For this review, take the finished solid that the model builds, in its own axes (mm). Face numbers are marked on the shaded views. A direction names the side the tool comes from. Coordinates: 2 decimals unless noted, no trailing zeros. Loops run counter-clockwise (first coordinate to the right, second up) from the corner with the lowest first, then second, coordinate; pieces in that order, holes last. Notation, with made-up numbers: (3.25, -38.75) - (42.25, -38.75) arc R20 ccw to (42.25, -6.75) - close; hole circle Ø11 at (86, -16). An arc over 180 degrees is marked (long way). Use one line per item in the form item = value. Start each with the question number.
1. Draft analysis for pull direction X (two halves, no side actions). For the marked faces 1, 2 and 3, state which applies: +X half, -X half, draft (parallel to the pull), parting line (faces both ways), or undercut.
2. For pin 1 Ø4.5 at (x, y) = (63, 0) entering from +Z; pin 2 Ø4 at (x, z) = (55.5, -1) entering from -Y; pin 3 Ø4 at (x, y) = (56.5, 2.5) entering from -Z, all flat-tipped, find the tip position at first contact; note any pin that passes through.
3. Add section B-B on x = 18. Give the boundary of the cut face in (y, z), and give its area (3 significant figures).
4. To check wall thickness, follow probe 1 along X at (y, z) = (0, 3.2); probe 2 along Z at (x, y) = (22.5, -5); probe 3 along X at (y, z) = (0, -1.25). State the ranges of each line that lie inside material, in increasing order.
5. Machinability: for the marked faces 4 and 5, which of the approach directions +Z, -Z, +X, -X, +Y, -Y give a long, thin tool a straight path to every point of the face, cutting with its end or side? Answer none if there is none.
6. Add section A-A on y = 0. Count the separate pieces of the cut face and the enclosed holes in it, and give its area (3 significant figures).
```python
from build123d import *

# Parameters (mm, degrees)
SKIZZE1_W                            = 63
SKIZZE1_H                            = 6
SKIZZE2_W                            = 18
SKIZZE2_H                            = 14
AUFSATZ_LINEAR_AUSTRAGEN1_DEPTH      = 9
SCHNITT_LINEAR_AUSTRAGEN1_DEPTH      = 72.909665553
SCHNITT_LINEAR_AUSTRAGEN1_DEPTH_BACK = 72.909665553
SKIZZE3_R                            = 2
SCHNITT_LINEAR_AUSTRAGEN2_DEPTH      = 72.909665553
SCHNITT_LINEAR_AUSTRAGEN2_DEPTH_BACK = 72.909665553
SKIZZE4_W                            = 15
SKIZZE4_H                            = 4
SCHNITT_LINEAR_AUSTRAGEN4_DEPTH      = 72.909665553
SCHNITT_LINEAR_AUSTRAGEN4_DEPTH_BACK = 72.909665553
SCHNITT_LINEAR_AUSTRAGEN5_DEPTH      = 5
SCHNITT_LINEAR_AUSTRAGEN5_DEPTH_BACK = 65.02343321
SKIZZE9_OUTSIDE_W                    = 32.83
SKIZZE9_OUTSIDE_H                    = 36.83
SKIZZE9_OUTSIDE_R                    = 6
SKIZZE11_W                           = 0.94
SKIZZE11_H                           = 2.5
SKIZZE14_W                           = 4
SKIZZE14_H                           = 3
SCHNITT_LINEAR_AUSTRAGEN7_DEPTH      = 45
FASE1_SIZE                           = 1
SCHNITT_LINEAR_START                 = -6.0000001
SCHNITT_LINEAR_AUSTRAGEN8_DEPTH      = 12.0000001
SCHNITT_LINEAR_AUSTRAGEN9_DEPTH      = 68.535176128
SCHNITT_LINEAR_AUSTRAGEN9_DEPTH_BACK = 68.535176128
SKIZZE16_W                           = 13.06
SKIZZE16_H                           = 1
VERRUNDUNG2_R                        = 2
VERRUNDUNG3_R                        = 2
VERRUNDUNG4_R                        = 2


with BuildPart() as part:
    # Skizze1 → Rotation1 (revolve)
    with BuildSketch(Plane.XY, mode=Mode.PRIVATE) as rotation1_sk:
        with Locations((21.5, 3)):
            Rectangle(SKIZZE1_W, SKIZZE1_H)
    revolve(rotation1_sk.sketch.rotate(Axis((0, 0, 0), (1, 0, 0)), 90), axis=Axis((0, 0, 0), (1, 0, 0)))

    # Skizze2 → Aufsatz-Linear austragen1 (add, symmetric)
    with BuildSketch(Plane(origin=(0, 0, 0), x_dir=(1, 0, 0), z_dir=(0, 1, 0))):
        with Locations((62, 0)):
            Rectangle(SKIZZE2_W, SKIZZE2_H)
    extrude(amount=AUFSATZ_LINEAR_AUSTRAGEN1_DEPTH, both=True)

    # Skizze3 → Schnitt-Linear austragen1 (cut, two sides: drawn at the far end of the back side and taken through both)
    with BuildSketch(Plane.XY.offset(-SCHNITT_LINEAR_AUSTRAGEN1_DEPTH_BACK)):
        with Locations((63, 0)):
            Circle(SKIZZE3_R)
    extrude(amount=SCHNITT_LINEAR_AUSTRAGEN1_DEPTH + SCHNITT_LINEAR_AUSTRAGEN1_DEPTH_BACK, mode=Mode.SUBTRACT)

    # Skizze4 → Schnitt-Linear austragen2 (cut, two sides: drawn at the far end of the back side and taken through both)
    with BuildSketch(Plane(origin=(0, 0, 0), x_dir=(1, 0, 0), z_dir=(0, 1, 0)).offset(-SCHNITT_LINEAR_AUSTRAGEN2_DEPTH_BACK)):
        with Locations((64.5, 0)):
            Rectangle(SKIZZE4_W, SKIZZE4_H)
    extrude(amount=SCHNITT_LINEAR_AUSTRAGEN2_DEPTH + SCHNITT_LINEAR_AUSTRAGEN2_DEPTH_BACK, mode=Mode.SUBTRACT)

    # Skizze7 → Schnitt-Linear austragen4 (cut, two sides: drawn at the far end of the back side and taken through both)
    with BuildSketch(Plane(origin=(0, 0, 0), x_dir=(1, 0, 0), z_dir=(0, 1, 0)).offset(-SCHNITT_LINEAR_AUSTRAGEN4_DEPTH_BACK)):
        Polygon((53, -5.5), (17, -3.580275313), (16.870966522, -6), (53, -6), align=None)
    extrude(amount=SCHNITT_LINEAR_AUSTRAGEN4_DEPTH + SCHNITT_LINEAR_AUSTRAGEN4_DEPTH_BACK, mode=Mode.SUBTRACT)

    # Skizze9 outside → Schnitt-Linear austragen5 (cut, two sides: drawn at the far end of the back side and taken through both)
    with BuildSketch(Plane.ZY.offset(-53).offset(-SCHNITT_LINEAR_AUSTRAGEN5_DEPTH_BACK)):
        Rectangle(SKIZZE9_OUTSIDE_W, SKIZZE9_OUTSIDE_H)
        Circle(SKIZZE9_OUTSIDE_R, mode=Mode.SUBTRACT)
    extrude(amount=SCHNITT_LINEAR_AUSTRAGEN5_DEPTH + SCHNITT_LINEAR_AUSTRAGEN5_DEPTH_BACK, mode=Mode.SUBTRACT)

    # Skizze11 → Schnitt-Rotation1 (revolve, cut)
    with BuildSketch(Plane.XY, mode=Mode.PRIVATE) as schnitt_rotation1_sk:
        with Locations((53.47, 4.75)):
            Rectangle(SKIZZE11_W, SKIZZE11_H)
    revolve(schnitt_rotation1_sk.sketch.rotate(Axis((0, 0, 0), (1, 0, 0)), 90), axis=Axis((0, 0, 0), (1, 0, 0)), mode=Mode.SUBTRACT)

    # Skizze14 → Schnitt-Linear austragen7 (cut)
    with BuildSketch(Plane(origin=(57, 0, 0), x_dir=(0, 0, -1), z_dir=(1, 0, 0))):
        with Locations((0, 6)):
            Rectangle(SKIZZE14_W, SKIZZE14_H)
        with Locations((0, -6)):
            Rectangle(SKIZZE14_W, SKIZZE14_H)
    extrude(amount=-SCHNITT_LINEAR_AUSTRAGEN7_DEPTH, mode=Mode.SUBTRACT)

    # Fase1
    fase1_edges = [part.edges().sort_by_distance(p)[0] for p in [
        (-10, 0, -6),
    ]]
    chamfer(fase1_edges, length=FASE1_SIZE)

    # Schnitt-Linear austragen8: read off the stored shape, not the designer's step
    # Schnitt-Linear austragen8 outline → Schnitt-Linear austragen8 (cut)
    with BuildSketch(Plane.XY.offset(SCHNITT_LINEAR_START)):
        with BuildLine():
            Line((53.94, 7), (53.94, 4.5))
            Line((53.94, 4.5), (57.44, 4.5))
            Line((57.44, 4.5), (63.347474122, 3.984879137))
            ThreePointArc((63.347474122, 3.984879137), (67, 0), (63.347474122, -3.984879137))
            Line((63.347474122, -3.984879137), (57.44, -4.5))
            Line((57.44, -4.5), (53.94, -4.5))
            Line((53.94, -4.5), (53.94, -7))
            Line((53.94, -7), (72, -7))
            Line((72, -7), (72, 7))
            Line((72, 7), (53.94, 7))
        make_face()
    extrude(amount=SCHNITT_LINEAR_AUSTRAGEN8_DEPTH, mode=Mode.SUBTRACT)

    # Skizze16 → Schnitt-Linear austragen9 (cut, two sides: drawn at the far end of the back side and taken through both)
    with BuildSketch(Plane(origin=(0, 0, 0), x_dir=(1, 0, 0), z_dir=(0, 1, 0)).offset(-SCHNITT_LINEAR_AUSTRAGEN9_DEPTH_BACK)):
        with Locations((60.47, 5.5)):
            Rectangle(SKIZZE16_W, SKIZZE16_H)
        with Locations((60.47, -5.5)):
            Rectangle(SKIZZE16_W, SKIZZE16_H)
    extrude(amount=SCHNITT_LINEAR_AUSTRAGEN9_DEPTH + SCHNITT_LINEAR_AUSTRAGEN9_DEPTH_BACK, mode=Mode.SUBTRACT)

    # Verrundung2
    verrundung2_edges = [part.edges().sort_by_distance(p)[0] for p in [
        (12, 5.078427125, 2),
        (12, 5.078427125, -2),
    ]]
    fillet(verrundung2_edges, radius=VERRUNDUNG2_R - 0.0001)  # a hair under: the kernel refuses the full size

    # Verrundung3
    verrundung3_edges = [part.edges().sort_by_distance(p)[0] for p in [
        (12, -5.078427125, 2),
        (12, -5.078427125, -2),
    ]]
    fillet(verrundung3_edges, radius=VERRUNDUNG3_R - 0.0001)  # a hair under: the kernel refuses the full size

    # Verrundung4
    verrundung4_edges = [part.edges().sort_by_distance(p)[0] for p in [
        (57, 0, -2),
        (57, 0, 2),
    ]]
    fillet(verrundung4_edges, radius=VERRUNDUNG4_R - 0.0001)  # a hair under: the kernel refuses the full size


solid = part.part
```
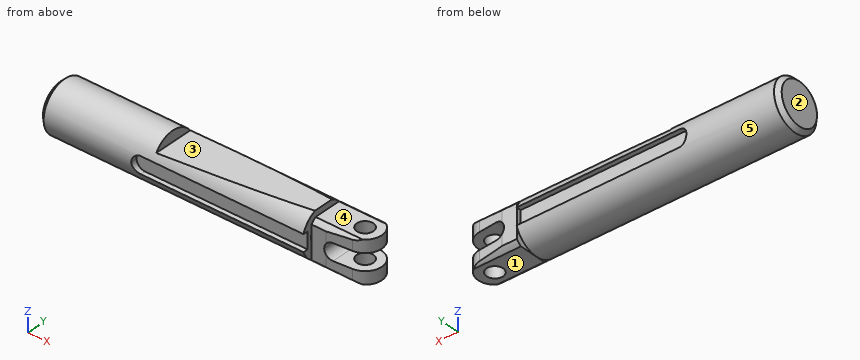
Conclusion:
q1.face_1 = draft
q1.face_2 = -X half
q1.face_3 = undercut
q2.pin_1 = 5
q2.pin_2 = -4.5
q2.pin_3 = -5
q3.outline = (-5.66, -2) arc R6 ccw to (5.66, -2) - (4.5, -2) - (4.5, 2) - (5.66, 2) arc R6 ccw to (4.77, 3.63) - (-4.77, 3.63) arc R6 ccw to (-5.66, 2) - (-4.5, 2) - (-4.5, -2) - close
q3.area = 86.2 mm^2
q4.probe_1 = -10 to 61, 65 to 67
q4.probe_2 = -3.32 to -2, 2 to 3.32
q4.probe_3 = -10 to 57.44
q5.face_4 = +Z, +X, +Y, -Y
q5.face_5 = +X, -X
q6.separate_pieces = 3
q6.enclosed_holes = 0
q6.area = 777 mm^2
